```python
from build123d import *

# Parameters (mm, degrees)
SKETCH1_W           = 20
SKETCH1_H           = 120
BOSS_EXTRUDE1_DEPTH = 20
CUT_EXTRUDE2_DEPTH  = 20
SKETCH5_W           = 18
SKETCH5_H           = 18
CUT_EXTRUDE4_DEPTH  = 120


with BuildPart() as part:
    # Sketch1 → Boss-Extrude1 (new body)
    with BuildSketch(Plane.XY):
        with Locations((6.772727273, -55.795454545)):
            Rectangle(SKETCH1_W, SKETCH1_H)
    extrude(amount=-BOSS_EXTRUDE1_DEPTH)

    # Sketch4 → Cut-Extrude2 (cut)
    with BuildSketch(Plane.ZY.offset(3.227272727)):
        Polygon((-20, 4.204545455), (0, -0.265984203), (0, 4.204545455), align=None)
    extrude(amount=-CUT_EXTRUDE2_DEPTH, mode=Mode.SUBTRACT)

    # Sketch5 → Cut-Extrude4 (cut)
    with BuildSketch(Plane.XZ.offset(115.795454545)):
        with Locations((7.772727273, -11)):
            Rectangle(SKETCH5_W, SKETCH5_H)
    extrude(amount=-CUT_EXTRUDE4_DEPTH, mode=Mode.SUBTRACT)


solid = part.part
```
Model file for the job. Use its own axes, mm. A direction names the side the tool comes from. Round coordinates to 2 decimals unless told otherwise and drop trailing zeros. Order: outer loops, then holes, each group sorted by start corner. A loop starts at its lowest first (then second) coordinate and runs counter-clockwise, first axis right, second up. Notation, with made-up numbers: (6.5, 40) -> (57.5, 40) arc R29 ccw to (57.5, 64) -> close; hole circle Ø10 at (22, 20). An arc over 180 degrees is marked (long way). Use one line per item in the form item = value.
Item 1: Flat gauge pins, fed straight in: pin 1 Ø4 at (x, y) = (1.5, -60.5) entering from +Z; pin 2 Ø5 at (y, z) = (-18.5, -12.5) entering from +X; pin 3 Ø5.5 at (x, y) = (7.5, -70.5) entering from -Z; pin 4 Ø6 at (x, z) = (1, -14) entering from +Y. Where does each tip first touch, or does it go through?
Returned:
pin_1 = 0
pin_2 = -1.23
pin_3 = -2
pin_4 = 3.31
Item 2: Drill centre lines: line 1 (Z direction, x = 4.5, y = -35); line 2 (X direction, y = -76.5, z = -13); line 3 (Y direction, x = 15, z = -1). Where is each one in solid material? Low to high.
Returned:
line_1 = -2 to 0
line_2 = -3.23 to -1.23
line_3 = -115.8 to -0.04
Item 3: Cut at B-B, the plane x = 10. Write the cut outline in (y, z), and give its area (3 significant figures).
Returned:
outline = (-115.8, -2) -> (0.18, -2) -> (-0.27, 0) -> (-115.8, 0) -> close
area = 232 mm^2
Item 4: Cut at A-A, the plane y = -54.5. Write the cut outline in (x, z).
Returned:
outline = (-3.23, -20) -> (-1.23, -20) -> (-1.23, -2) -> (16.77, -2) -> (16.77, 0) -> (-3.23, 0) -> close
Item 5: Tool access for faces 1 (the face through (8, -59, -2)), 2 (the face through (16.773, -59, -1)): list every direction of +Z, -Z, +X, -X, +Y, -Y with a clear straight run to the whole face (end or side of a thin tool).
Returned:
face_1 = -Z, +X, +Y, -Y
face_2 = +Z, -Z, +X, +Y, -Y
